Model file for the job. Use its own axes, mm. A direction names the side the tool comes from. Give positions to 0.01 mm unless a question says otherwise; leave off trailing zeros. Loops run counter-clockwise (first coordinate to the right, second up) from the corner with the lowest first, then second, coordinate; pieces in that order, holes last. Notation, with made-up numbers: M 74,22 L 120,22 A25 cw 120,38 Z; hole C 73,-4.5 d9. An arc over 180 degrees is marked long. Answer in a Markdown table with one row per item.
```python
from build123d import *

# Parameters (mm, degrees)
CHAMFER1_SIZE      = 0.25
CHAMFER2_SIZE      = 0.25
CHAMFER3_SIZE      = 0.25
SKETCH2_R          = 2.55
CUT_EXTRUDE1_DEPTH = 15


with BuildPart() as part:
    # Sketch1 → Revolve1 (revolve)
    with BuildSketch(Plane.XY, mode=Mode.PRIVATE) as revolve1_sk:
        with BuildLine():
            Line((17.5, 15), (17.5, 158))
            ThreePointArc((17.5, 158), (18.964466094, 161.535533906), (22.5, 163))
            Line((22.5, 163), (27.1, 163))
            Line((27.1, 163), (27.1, 180))
            Line((27.1, 180), (17, 180))
            Line((17, 180), (17, 177))
            Line((17, 177), (14, 177))
            Line((14, 177), (14, 197.5))
            Line((14, 197.5), (11.5, 200))
            Line((11.5, 200), (0, 200))
            Line((0, 200), (0, 0))
            Line((0, 0), (11.226497308, 0))
            Line((11.226497308, 0), (17, 10))
            Line((17, 10), (17, 15))
            Line((17, 15), (17.5, 15))
        make_face()
    revolve(revolve1_sk.sketch.rotate(Axis((0, 0, 0), (0, 1, 0)), 90), axis=Axis((0, 0, 0), (0, 1, 0)))  # turned: the seam where the file's is

    # Chamfer1
    chamfer1_edges = [part.edges().sort_by_distance(p)[0] for p in [
        (0, 180, 27.1),
    ]]
    chamfer(chamfer1_edges, length=CHAMFER1_SIZE)

    # Chamfer2
    chamfer2_edges = [part.edges().sort_by_distance(p)[0] for p in [
        (0, 163, 27.1),
    ]]
    chamfer(chamfer2_edges, length=CHAMFER2_SIZE)

    # Chamfer3
    chamfer3_edges = [part.edges().sort_by_distance(p)[0] for p in [
        (0, 180, 17),
    ]]
    chamfer(chamfer3_edges, length=CHAMFER3_SIZE)

    # Sketch2 → Cut-Extrude1 (cut, symmetric)
    with BuildSketch(Plane.XY):
        with Locations((0, 189.875)):
            Circle(SKETCH2_R)
    extrude(amount=CUT_EXTRUDE1_DEPTH, both=True, mode=Mode.SUBTRACT)


solid = part.part
```
(1) Mould opens along Z. For faces 4 (the flat face through (-13, 177, 6)), 5 (the flat face through (0, 200, 0)), 6 (the cylindrical face through (-16.855, 12.535, 2.213)) say: pulls with the +Z half, pulls with the -Z half, needs draft (parallel to the pull), parting line crosses it, or undercut.
Established:
| item | result |
|---|---|
| face 4 | undercut |
| face 5 | needs draft |
| face 6 | parting line crosses it |
(2) Flat gauge pins, fed straight in: P1, Ø6.5, axis at x = 0, y = 189.875, coming from the +Z side; P2, Ø6, axis at y = 82.5, z = -17.5, coming from the +X side; P3, Ø10.5, axis at x = -7.5, z = -4, coming from the -Y side; P4, Ø5, axis at x = 4, z = -18, coming from the -Y side. Where does each tip first touch, or does it go through?
Established:
| item | result |
|---|---|
| P1 | stops at z = 14 |
| P2 | stops at x = 9.8 |
| P3 | stops at y = 0 |
| P4 | stops at y = 8.16 |
(3) Saw through at A-A, the plane y = 47.5. Give the cut face in (x, z).
Established:
| item | result |
|---|---|
| outline | C 0,0 d35 |
(4) Wall check: L1, parallel to X at y = 179, z = 0; L2, parallel to Y at x = 0, z = 7.25 (3 decimals); L3, parallel to Y at x = 21.5, z = -5.5. Give the ranges that are in metal, low to high.
Established:
| item | result |
|---|---|
| L1 | x = -27.1 to -17, -14 to 14, 17 to 27.1 |
| L2 | y = 0 to 187.325, 192.425 to 200 |
| L3 | y = 162.99 to 180 |
(5) Which spindle directions (+Z, -Z, +X, -X, +Y, -Y) get a long thin tool onto all of the face, cutting with end or side? Do faces 1 (the flat face through (-17, 15, -3)), 2 (the flat face through (0, 0, 0)), 3 (the cylindrical face through (5.362, 187.394, -12.932)). Say none if no direction does.
Established:
| item | result |
|---|---|
| face 1 | -Y |
| face 2 | +Z, -Z, +X, -X, -Y |
| face 3 | +Y |
